Part model, mm, in its own coordinate system. A direction names the side the tool comes from. Give positions to 0.01 mm unless a question says otherwise; leave off trailing zeros. Order: outer loops, then holes, each group sorted by start corner. A loop starts at its lowest first (then second) coordinate and runs counter-clockwise, first axis right, second up. Notation, with made-up numbers: M -22,-23 L -6,-23 A30 cw -6,13 Z; hole C 61,70 d11. An arc over 180 degrees is marked long. Answer as a JSON object with one key per item and string values.
from build123d import *

# Parameters (mm, degrees)
F1_DEPTH = 150
F2_R     = 2.55
F3_DEPTH = 15
F4_R     = 2


with BuildPart() as f1:
    # F0 (on Front) → F1 (new body)
    with BuildSketch(Plane.XZ):
        Polygon((-53.166667, 15), (-53.166667, 0), (46.833333, 0), (46.833333, 15), (4.333333, 15), (4.333333, 35), (-10.666667, 35), (-10.666667, 15), align=None)
    extrude(amount=F1_DEPTH)

    # F2 (on face) → F3 (cut, through all)
    with BuildSketch(Plane.YZ.offset(4.333333)):
        with Locations((-120, 27)):
            Circle(F2_R)
        with Locations((-30, 27)):
            Circle(F2_R)
    extrude(amount=-F3_DEPTH, mode=Mode.SUBTRACT)

    # F4
    f4_edges = [f1.edges().sort_by_distance(p)[0] for p in [
        (-10.666667, -75, 15),
        (4.333333, -75, 15),
    ]]
    fillet(f4_edges, radius=F4_R)


solid = f1.part
1. Cut at D-D on x = -35. Give the cut face in (y, z).
Worked answers:
{"outline": "M -150,0 L 0,0 L 0,15 L -150,15 Z"}
2. Pin check, flat tips, straight feed: P1, Ø5.5, axis at y = -98, z = 29.5, coming from the -X side; P2, Ø20, axis at x = 29.5, y = -89, coming from the +Z side; P3, Ø1.5, axis at y = -93, z = 23.5, coming from the +X side. Stop position of each tip, or through.
Worked answers:
{"P1": "stops at x = -10.67", "P2": "stops at z = 15", "P3": "stops at x = 4.33"}
3. Two-plate mould, pull along Y, no slides. Class faces 1 (the flat face through (-3, -74, 35)), 2 (the flat face through (-4, 0, 10)), 3 (the cylindrical face through (-3.062, -32.548, 27.112)): +Y half, -Y half, draft (parallel to the pull), parting line (faces both ways), or undercut.
Worked answers:
{"face 1": "draft", "face 2": "+Y half", "face 3": "undercut"}
4. Cut at A-A on y = -30. Give the cut face in (x, z).
Worked answers:
{"outline": "M -53.17,0 L 46.83,0 L 46.83,15 L 6.33,15 A2 cw 4.33,17 L 4.33,24.45 L -10.67,24.45 L -10.67,17 A2 cw -12.67,15 L -53.17,15 Z; M -10.67,29.55 L 4.33,29.55 L 4.33,35 L -10.67,35 Z"}
5. Cut at B-B on z = 27. Give the cut face in (x, y), plus the area to 3 significant figures.
Worked answers:
{"outline": "M -10.67,-150 L 4.33,-150 L 4.33,-122.55 L -10.67,-122.55 Z; M -10.67,-117.45 L 4.33,-117.45 L 4.33,-32.55 L -10.67,-32.55 Z; M -10.67,-27.45 L 4.33,-27.45 L 4.33,0 L -10.67,0 Z", "area": "2,100 mm^2"}
6. Which spindle directions (+Z, -Z, +X, -X, +Y, -Y) get a long thin tool onto all of the face, cutting with end or side? Do faces 4 (the flat face through (-10.667, -74, 26)), 5 (the flat face through (-4, -74, 0)), 6 (the flat face through (4.333, -74, 26)). Say none if no direction does.
Worked answers:
{"face 4": "+Z, -X, +Y, -Y", "face 5": "-Z, +X, -X, +Y, -Y", "face 6": "+Z, +X, +Y, -Y"}
7. Probe line 1 along Z through (x, y) = (1, -30); line 2 along Z through (x, y) = (34, -128); line 3 along X through (y, z) = (-134, 32). List the from-to ranges inside material, lowest first.
Worked answers:
{"line 1": "z = 0 to 24.45, 29.55 to 35", "line 2": "z = 0 to 15", "line 3": "x = -10.67 to 4.33"}
8. Cut at C-C on y = -104.5. Give the cut face in (x, z).
Worked answers:
{"outline": "M -53.17,0 L 46.83,0 L 46.83,15 L 6.33,15 A2 cw 4.33,17 L 4.33,35 L -10.67,35 L -10.67,17 A2 cw -12.67,15 L -53.17,15 Z"}
